Design review of the part shown in the three views and the two pictorial views. Dimensions are in mm from the part's minimum x, y and z. Round coordinates to 2 decimals unless told otherwise and drop trailing zeros. Loops run counter-clockwise (first coordinate to the right, second up) from the corner with the lowest first, then second, coordinate; pieces in that order, holes last. Notation, with made-up numbers: M 5,-27 L 11,-27 A27 cw 11,-8 Z; hole C 6.25,43.25 d2. An arc over 180 degrees is marked long. Answer as CSV lines item,"result". Start each with the question number.
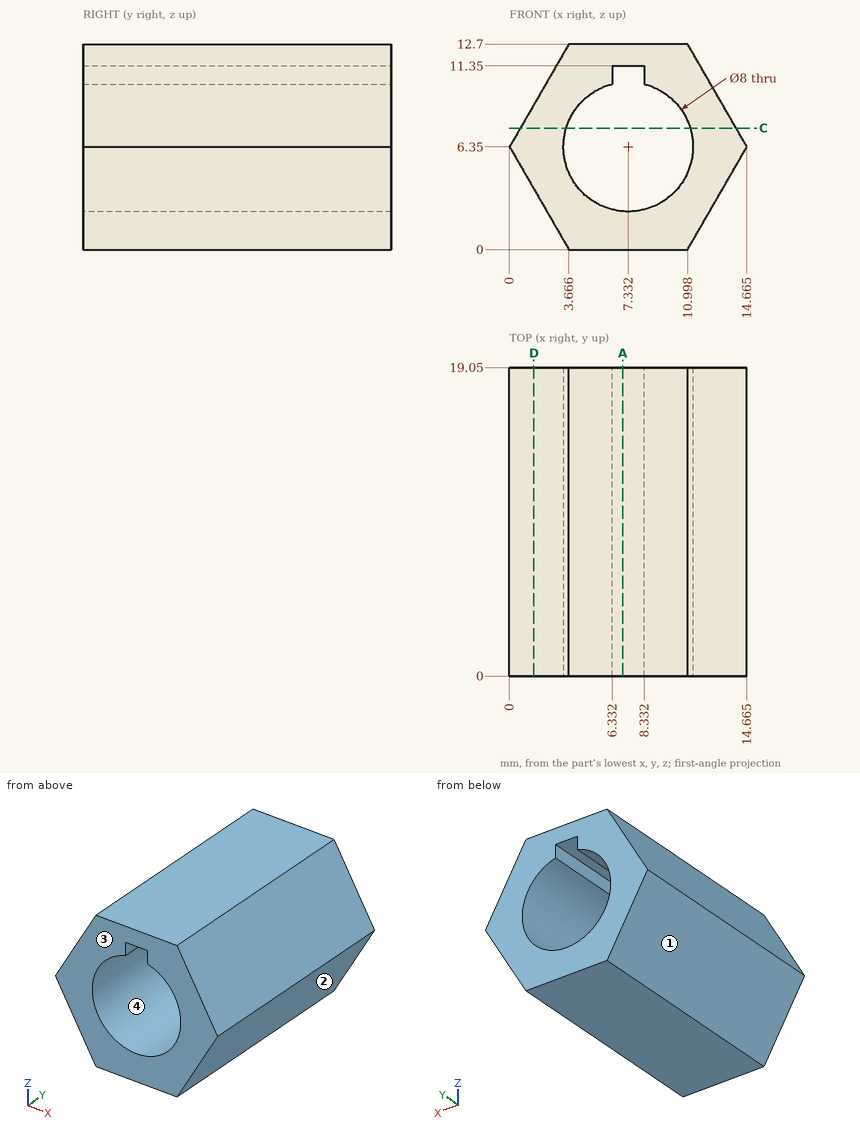
Item 1: The part is to be moulded in two halves that separate along X. For the marked faces 1, 2, 3 and 4, say which applies: +X half, -X half, draft (parallel to the pull), parting line (faces both ways), or undercut.
Item 2: Consider section A-A, the plane x = 7. Write out the cut boundary in (y, z).
Item 3: Consider section C-C, the plane z = 7.5. Write out the cut boundary in (x, y).
Item 4: Insertion check: pin 1 Ø0.6 at (y, z) = (8, 10.5) entering from -X; pin 2 Ø0.9 at (y, z) = (8, 11) entering from +X; pin 3 Ø6 at (y, z) = (11.5, 10) entering from +X. Each pin has a flat end and moves straight along its axis. Give the tip position at first contact, or say it passes through.
Item 5: Consider section D-D, the plane x = 1.5. Write out the cut boundary in (y, z).
Item 6: To check wall thickness, follow line 1 (X direction, y = 1.75, z = 6) (1 decimal); line 2 (Z direction, x = 10.5, y = 16.5) (1 decimal); line 3 (X direction, y = 9.75, z = 5.75) (1 decimal). State the ranges of each line that lie inside material, in increasing order.
Found:
1,face 1,"-X half"
1,face 2,"+X half"
1,face 3,"draft"
1,face 4,"undercut"
2,outline,"M 0,0 L 19.05,0 L 19.05,2.36 L 0,2.36 Z; M 0,11.35 L 19.05,11.35 L 19.05,12.7 L 0,12.7 Z"
3,outline,"M 0.66,0 L 3.5,0 L 3.5,19.05 L 0.66,19.05 Z; M 11.16,0 L 14,0 L 14,19.05 L 11.16,19.05 Z"
4,pin 1,"stops at x = 2.22"
4,pin 2,"stops at x = 12.24"
4,pin 3,"stops at x = 14.29"
5,outline,"M 0,3.75 L 19.05,3.75 L 19.05,8.95 L 0,8.95 Z"
6,line 1,"x = 0.2 to 3.3, 11.3 to 14.5"
6,line 2,"z = 0 to 3.9, 8.8 to 12.7"
6,line 3,"x = 0.3 to 3.4, 11.3 to 14.3"
